Geometry: final body of the model. Coordinates: model frame, mm. A direction names the side the tool comes from. Give positions to 0.01 mm unless a question says otherwise; leave off trailing zeros. Write each loop counter-clockwise with the first axis right and the second up, starting at its lowest first coordinate (ties: lowest second). Pieces come first, ordered by that corner, then holes. Notation, with made-up numbers: (82.25, 69.25) -> (138.25, 69.25) arc R11 cw to (138.25, 75.25) -> close; hole circle Ø9 at (-19.75, 39). An arc over 180 degrees is marked (long way). Answer in a Markdown table with one row per item. Add a question column.
Item 1: Section query C-C on x = 0. Output: boundary loops of the cut face in (y, z) (1 decimal).
Item 2: Section query B-B on z = 1.5. Output: boundary loops of the cut face in (x, y), plus the area to 3 significant figures.
Item 3: First-contact query: P1, Ø1.5, axis at x = 0, y = -2.5, coming from the +Z side; P2, Ø8, axis at x = -1.5, z = 9.5, coming from the +Y side. Flat tips, straight axial feed; report the tip coordinate or a pass-through.
Item 4: Draft query along Z for faces 4 (the flat face through (5, 0, 6)), 5 (the flat face through (-5.47, -2.5, 8.9)), 6 (the flat face through (1.57, -2.5, 11.18)). Return one class per face: +Z half, -Z half, draft (parallel to the pull), parting line (faces both ways), or undercut.
Item 5: Access query for faces 1 (the flat face through (-1.52, -2.5, 10.81)), 2 (the flat face through (4.74, -2.5, 10.65)), 3 (the cylindrical face through (-0.202, -2.504, -9.205)). Directions: +Z, -Z, +X, -X, +Y, -Y. A direction counts if a zero-diameter tool reaches every point of the face in a straight line with its end or side. Return the directions, or none.
Item 6: Section query A-A on y = -0.3. Output: boundary loops of the cut face in (x, z) (1 decimal).
Item 7: Material intervals for probe 1 along X at (y, z) = (-1.2, 8.25); probe 2 along Z at (x, y) = (4.75, -1.55); probe 3 along Z at (x, y) = (0, -2.95) (1 decimal), sorted ascending. Write a range as from..to.
Item 8: Section query D-D on x = -8. Output: boundary loops of the cut face in (y, z).
```python
from build123d import *

# Parameters (mm, degrees)
F0_R     = 6.985
F1_DEPTH = 5.08


with BuildPart() as f1:
    # F0 (on Front) → F1 (new body)
    with BuildSketch(Plane.XZ):
        with BuildLine():
            ThreePointArc((-9.2075, 0), (0, 9.2075), (9.2075, 0))
            Line((9.2075, 0), (10.355688, 6.985))
            Line((10.355688, 6.985), (10.773211, 9.525))
            Line((10.773211, 9.525), (6.530722, 7.783012))
            Line((6.530722, 7.783012), (8.979743, 10.701641))
            Line((8.979743, 10.701641), (4.132444, 9.281622))
            Line((4.132444, 9.281622), (5.372178, 12.066108))
            Line((5.372178, 12.066108), (1.413999, 10.061124))
            Line((1.413999, 10.061124), (1.732148, 12.324876))
            Line((1.732148, 12.324876), (-1.413999, 10.061124))
            Line((-1.413999, 10.061124), (-1.626099, 11.570292))
            Line((-1.626099, 11.570292), (-4.132444, 9.281622))
            Line((-4.132444, 9.281622), (-4.442378, 9.977743))
            Line((-4.442378, 9.977743), (-6.530722, 7.783012))
            Line((-6.530722, 7.783012), (-10.773211, 9.525))
            Line((-10.773211, 9.525), (-10.355688, 6.985))
            Line((-10.355688, 6.985), (-9.2075, 0))
        make_face()
        with BuildLine():
            ThreePointArc((-9.2075, 0), (0, -9.2075), (9.2075, 0))
            ThreePointArc((9.2075, 0), (0, 9.2075), (-9.2075, 0))
        make_face()
        Circle(F0_R, mode=Mode.SUBTRACT)
    extrude(amount=F1_DEPTH)


solid = f1.part
```
Findings below:
| question | item | result |
|---|---|---|
| 1 | outline | (-5.1, -9.2) -> (0, -9.2) -> (0, -7) -> (-5.1, -7) -> close; (-5.1, 7) -> (0, 7) -> (0, 11.1) -> (-5.1, 11.1) -> close |
| 2 | outline | (-9.45, -5.08) -> (-6.82, -5.08) -> (-6.82, 0) -> (-9.45, 0) -> close; (6.82, -5.08) -> (9.45, -5.08) -> (9.45, 0) -> (6.82, 0) -> close |
| 2 | area | 26.7 mm^2 |
| 3 | P1 | stops at z = 11.62 |
| 3 | P2 | stops at y = 0 |
| 4 | face 4 | draft |
| 4 | face 5 | +Z half |
| 4 | face 6 | undercut |
| 5 | face 1 | +Z, +Y, -Y |
| 5 | face 2 | +Y, -Y |
| 5 | face 3 | -Z, +Y, -Y |
| 6 | outline | (-10.8, 9.5) -> (-9.2, 0) arc R9.2 ccw to (9.2, 0) -> (10.8, 9.5) -> (6.5, 7.8) -> (9, 10.7) -> (4.1, 9.3) -> (5.4, 12.1) -> (1.4, 10.1) -> (1.7, 12.3) -> (-1.4, 10.1) -> (-1.6, 11.6) -> (-4.1, 9.3) -> (-4.4, 10) -> (-6.5, 7.8) -> close; hole circle Ø14 at (0, 0) |
| 7 | probe 1 | x = -10.56..-7.67, -6.09..6.92, 7.67..10.56 |
| 7 | probe 2 | z = -7.89..-5.12, 5.12..9.46, 10.67..11.75 |
| 7 | probe 3 | z = -9.2..-7, 7..11.1 |
| 8 | outline | (-5.08, -4.56) -> (0, -4.56) -> (0, 8.39) -> (-5.08, 8.39) -> close |
